from build123d import *

# Parameters (mm, degrees)
F1_DEPTH = 5
F2_DEPTH = 25


with BuildPart() as f1:
    # F0 (on Top) → F1 (new body)
    with BuildSketch(Plane.XY):
        Polygon((-21, 21), (-21, 0), (-21, -21), (21, -21), (21, 21), align=None)
        with BuildLine():
            ThreePointArc((-20, 0), (0, 20), (20, 0))
            ThreePointArc((20, 0), (0, -20), (-20, 0))
        make_face(mode=Mode.SUBTRACT)
        with BuildLine():
            ThreePointArc((-20, 0), (0, -20), (20, 0))
            ThreePointArc((20, 0), (0, 20), (-20, 0))
        make_face()
    extrude(amount=F1_DEPTH)

    # F0 (on Top) → F2 (join)
    with BuildSketch(Plane.XY):
        Polygon((-21, 21), (-21, 0), (-21, -21), (21, -21), (21, 21), align=None)
        with BuildLine():
            ThreePointArc((-20, 0), (0, 20), (20, 0))
            ThreePointArc((20, 0), (0, -20), (-20, 0))
        make_face(mode=Mode.SUBTRACT)
    extrude(amount=F2_DEPTH)


solid = f1.part
Source: CAD feature listing. Evaluate the final solid. Frame: model axes, mm. A direction names the side the tool comes from. Round coordinates to 2 decimals unless told otherwise and drop trailing zeros. Write each loop counter-clockwise with the first axis right and the second up, starting at its lowest first coordinate (ties: lowest second). Pieces come first, ordered by that corner, then holes. Notation, with made-up numbers: M 9,55 L 16,55 A12 ccw 16,76 Z; hole C 87,-14 d8. An arc over 180 degrees is marked long. One line per item, written item: value. Start each with the question number.
Item 1: Ray query, L1, parallel to Y at x = 0, z = 18.5; L2, parallel to Z at x = -7.5, y = -8.5; L3, parallel to Y at x = -5, z = 17.5. Return the intervals inside material, ascending. Write a range as from..to.
Item 2: Section query C-C (z = 21.25). Return the cut outline in (x, y).
Item 3: Set-up query: faces 1 (the flat face through (0, 0, 5)), 2 (the flat face through (0, 0, 0)). Return all of +Z, -Z, +X, -X, +Y, -Y with unobstructed straight access to the full face (end or side cutting, diameter ignored); none if empty.
Item 4: Mould query, pull axis X, two halves, no side actions, for faces 3 (the flat face through (0, 21, 12)), 4 (the cylindrical face through (-16, 12, 15)), 5 (the flat face through (21, 0, 12)). Classes: pulls with the +X half, pulls with the -X half, needs draft (parallel to the pull), parting line crosses it, or undercut.
Item 5: Pin query (flat end, axial travel): pin 1 (6 mm diameter, centred on x = 2.5, y = -10.5, fed in from -Z); pin 2 (1.5 mm diameter, centred on x = 9, y = -2, fed in from +Z). Return the tip coordinate at first contact, or that it passes through.
Item 6: Section query A-A (y = 0). Return the cut outline in (x, z), plus the area to 3 significant figures.
Result set:
1. L1: y = -21..-20, 20..21
1. L2: z = 0..5
1. L3: y = -21..-19.36, 19.36..21
2. outline: M -21,-21 L 21,-21 L 21,21 L -21,21 Z; hole C 0,0 d40
3. face 1: +Z
3. face 2: -Z, +X, -X, +Y, -Y
4. face 3: needs draft
4. face 4: undercut
4. face 5: pulls with the +X half
5. pin 1: stops at z = 0
5. pin 2: stops at z = 5
6. outline: M -21,0 L 21,0 L 21,25 L 20,25 L 20,5 L -20,5 L -20,25 L -21,25 Z
6. area: 250 mm²
